from build123d import *

# Parameters (mm, degrees)
SKETCH1_R           = 8.33
BOSS_EXTRUDE1_DEPTH = 7.16
SKETCH2_R           = 3.5
BOSS_EXTRUDE2_DEPTH = 22.13
SKETCH3_W           = 15
SKETCH3_H           = 11.20454244
BOSS_EXTRUDE3_DEPTH = 1.2
BOSS_EXTRUDE4_START = -0.2
SKETCH4_W           = 1.15
SKETCH4_H           = 4.9
BOSS_EXTRUDE4_DEPTH = 0.6
LPATTERN1_COUNT     = 2
LPATTERN1_PITCH     = 5
LPATTERN1_COL_COUNT = 2
LPATTERN1_COL_PITCH = 5


with BuildPart() as part:
    # Sketch1 → Boss-Extrude1 (new body)
    with BuildSketch(Plane.XY):
        Circle(SKETCH1_R)
    extrude(amount=BOSS_EXTRUDE1_DEPTH)

    # Sketch2 → Boss-Extrude2 (add)
    with BuildSketch(Plane.XY.offset(7.16)):
        Circle(SKETCH2_R)
    extrude(amount=BOSS_EXTRUDE2_DEPTH)

    # Sketch3 → Boss-Extrude3 (add)
    with BuildSketch(Plane.XY.offset(7.16)):
        with Locations((0, -6.09772878)):
            Rectangle(SKETCH3_W, SKETCH3_H)
    extrude(amount=-BOSS_EXTRUDE3_DEPTH)

    # Sketch4 → Boss-Extrude4 (add)
    with BuildSketch(Plane(origin=(0, 0, 5.96), x_dir=(-1, 0, 0), z_dir=(0, 0, -1)).offset(BOSS_EXTRUDE4_START)):
        with Locations((0, -14.15)):
            Rectangle(SKETCH4_W, SKETCH4_H)
    boss_extrude4 = extrude(amount=BOSS_EXTRUDE4_DEPTH)

    # LPattern1: Boss-Extrude4 ×2
    with Locations(*[(i * LPATTERN1_PITCH, 0, 0) for i in range(1, LPATTERN1_COUNT)]):
        add(boss_extrude4)

    # LPattern1 col: Boss-Extrude4 ×2
    with Locations(*[(-i * LPATTERN1_COL_PITCH, 0, 0) for i in range(1, LPATTERN1_COL_COUNT)]):
        add(boss_extrude4)


solid = part.part
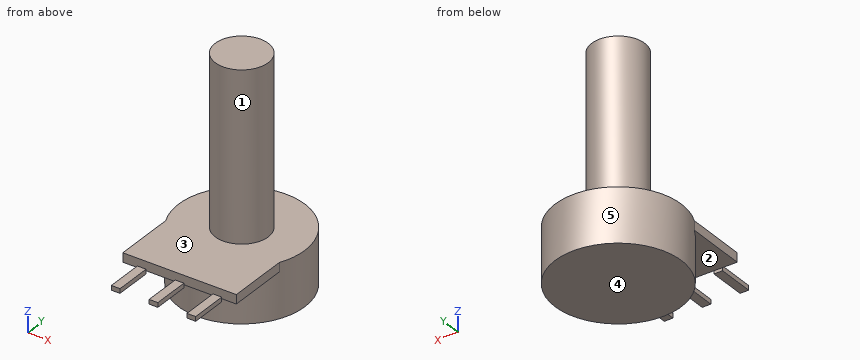
Can you work these out from the model? Positions are in its coordinate system, mm. Face numbers are marked on the shaded views. A direction names the side the tool comes from. Give positions to 0.01 mm unless a question says otherwise; leave off trailing zeros. Order: outer loops, then holes, each group sorted by start corner. A loop starts at its lowest first (then second) coordinate and runs counter-clockwise, first axis right, second up. Notation, with made-up numbers: M 71.5,-20 L 89.5,-20 A25 cw 89.5,15 Z; hole C -39,-37.75 d10. An arc over 180 degrees is marked long. Use a Markdown table: item, result. Add a question column.
Item 1: Will these pins go through, and if not, where does the flat tip stop? pin 1 (0.7 mm diameter, centred on y = -14, z = 6, fed in from -X) (3 decimals); pin 2 (8 mm diameter, centred on x = -2, z = 16, fed in from +Y); pin 3 (1.3 mm diameter, centred on x = 5, y = -14, fed in from -Z); pin 4 (1.5 mm diameter, centred on y = 5.5, z = 20.5, fed in from +X).
Item 2: If I drill on L1, parallel to Z at x = -3.25, y = 6; L2, parallel to Z at x = 0, y = -9; L3, parallel to Y at x = -2, z = 26, over which ranges is the centre line in solid material (lowest first)? Write a range as [from, to].
Item 3: Suppose I cut it at A-A (y = -13.5). List the corners of the cut face in (x, z) for me (3 decimals).
Item 4: Suppose I cut it at B-B (x = 0). List the corners of the cut face in (y, z) for me.
Item 5: For the marked faces 4 and 5, which set-ups out of +Z, -Z, +X, -X, +Y, -Y let a thin tool reach every point of the face, with its end or its side?
Item 6: Suppose I cut it at D-D (z = 4.5). List the corners of the cut face in (x, y) for me.
Item 7: We'd pull the mould along Y, two halves only. Please class the marked faces 1, 2 and 3: +Y half, -Y half, draft (parallel to the pull), parting line (faces both ways), or undercut.
Item 8: Suppose I cut it at C-C (y = 0). List the corners of the cut face in (x, z) for me.
Answer sheet:
| question | item | result |
|---|---|---|
| 1 | pin 1 | stops at x = -5.575 |
| 1 | pin 2 | stops at y = 3.5 |
| 1 | pin 3 | stops at z = 5.56 |
| 1 | pin 4 | passes through |
| 2 | L1 | z = [0, 7.16] |
| 2 | L2 | z = [5.96, 7.16] |
| 2 | L3 | y = [-2.87, 2.87] |
| 3 | outline | M -5.575,5.56 L -4.425,5.56 L -4.425,6.16 L -5.575,6.16 Z; M -0.575,5.56 L 0.575,5.56 L 0.575,6.16 L -0.575,6.16 Z; M 4.425,5.56 L 5.575,5.56 L 5.575,6.16 L 4.425,6.16 Z |
| 4 | outline | M -16.6,5.56 L -11.7,5.56 L -11.7,5.96 L -8.33,5.96 L -8.33,0 L 8.33,0 L 8.33,7.16 L 3.5,7.16 L 3.5,29.29 L -3.5,29.29 L -3.5,7.16 L -11.7,7.16 L -11.7,6.16 L -16.6,6.16 Z |
| 5 | face 4 | -Z, +X, -X, +Y, -Y |
| 5 | face 5 | -Z |
| 6 | outline | C 0,0 d16.66 |
| 7 | face 1 | parting line |
| 7 | face 2 | undercut |
| 7 | face 3 | draft |
| 8 | outline | M -8.33,0 L 8.33,0 L 8.33,7.16 L 3.5,7.16 L 3.5,29.29 L -3.5,29.29 L -3.5,7.16 L -8.33,7.16 Z |
